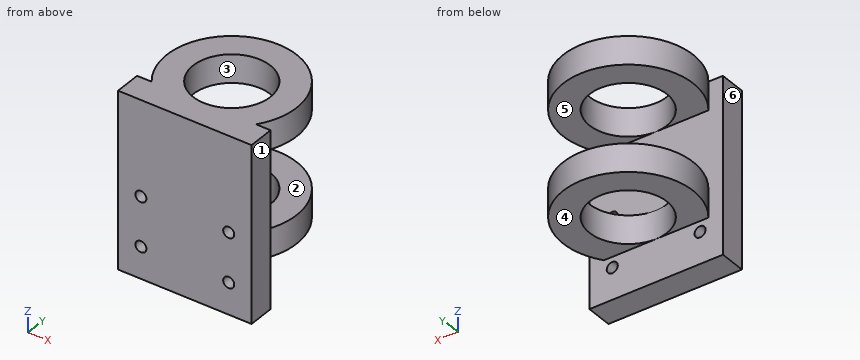
```python
from build123d import *

# Parameters (mm, degrees)
ESQUISSE1_R                = 18.5
ESQUISSE1_R_2              = 11
BOSS_EXTRU_19_DEPTH        = 8
BOSS_EXTRU_20_DEPTH        = 30
BOSS_EXTRU_20_DEPTH_BACK   = 20
R_P_TITION_LIN_AIRE1_COUNT = 2
R_P_TITION_LIN_AIRE1_PITCH = 30
ENL_V_MAT_EXTRU_1_REACH    = 48.165
ESQUISSE8_R                = 1.575


with BuildPart() as part:
    # Esquisse1 → Boss.-Extru.19 (new body)
    with BuildSketch(Plane.XY):
        Circle(ESQUISSE1_R)
        Circle(ESQUISSE1_R_2, mode=Mode.SUBTRACT)
    boss_extru_19 = extrude(amount=-BOSS_EXTRU_19_DEPTH)

    # Esquisse1_5 → Boss.-Extru.20 (add, two sides: drawn at the far end of the back side and taken through both)
    with BuildSketch(Plane.XY.offset(-BOSS_EXTRU_20_DEPTH_BACK)):
        with BuildLine():
            ThreePointArc((14.874474781, -11), (8.329165624, -16.518928537), (0, -18.5))
            Line((0, -18.5), (19, -18.5))
            Line((19, -18.5), (19, -11))
            Line((19, -11), (14.874474781, -11))
        make_face()
        with BuildLine():
            Line((-19, -18.5), (0, -18.5))
            ThreePointArc((0, -18.5), (-8.329165624, -16.518928537), (-14.874474781, -11))
            Line((-14.874474781, -11), (-19, -11))
            Line((-19, -11), (-19, -18.5))
        make_face()
        with BuildLine():
            Line((0, -11), (0, -11.058417443))
            Line((0, -11.058417443), (0, -18.5))
            ThreePointArc((0, -18.5), (8.329165624, -16.518928537), (14.874474781, -11))
            Line((14.874474781, -11), (1.4e-08, -11))
        make_face()
        with BuildLine():
            Line((0, -18.5), (0, -11.058417443))
            Line((0, -11.058417443), (0, -11))
            Line((1.4e-08, -11), (-14.874474781, -11))
            ThreePointArc((-14.874474781, -11), (-8.329165624, -16.518928537), (0, -18.5))
        make_face()
    extrude(amount=BOSS_EXTRU_20_DEPTH + BOSS_EXTRU_20_DEPTH_BACK)

    # R_p_tition lin_aire1: Boss.-Extru.19 ×2
    with Locations(*[(0, 0, i * R_P_TITION_LIN_AIRE1_PITCH) for i in range(1, R_P_TITION_LIN_AIRE1_COUNT)]):
        add(boss_extru_19)

    # Esquisse8 → Enl_v. mat.-Extru.1 (cut, up to next)
    with BuildSketch(Plane(origin=(0, -11, 0), x_dir=(1, 0, 0), z_dir=(0, 1, 0)), mode=Mode.PRIVATE) as enl_v_mat_extru_1_sk1:
        with Locations(Location((-12.5, 11, 0), (0, 0, 270))):
            Circle(ESQUISSE8_R)
    enl_v_mat_extru_1_tool1 = extrude(enl_v_mat_extru_1_sk1.sketch, amount=-ENL_V_MAT_EXTRU_1_REACH, mode=Mode.PRIVATE) & part.part
    # Esquisse8 → Enl_v. mat.-Extru.1 (cut, up to next)
    with BuildSketch(Plane(origin=(0, -11, 0), x_dir=(1, 0, 0), z_dir=(0, 1, 0)), mode=Mode.PRIVATE) as enl_v_mat_extru_1_sk2:
        with Locations(Location((12.5, 11, 0), (0, 0, 90))):
            Circle(ESQUISSE8_R)
    enl_v_mat_extru_1_tool2 = extrude(enl_v_mat_extru_1_sk2.sketch, amount=-ENL_V_MAT_EXTRU_1_REACH, mode=Mode.PRIVATE) & part.part
    # Esquisse8 → Enl_v. mat.-Extru.1 (cut, up to next)
    with BuildSketch(Plane(origin=(0, -11, 0), x_dir=(1, 0, 0), z_dir=(0, 1, 0)), mode=Mode.PRIVATE) as enl_v_mat_extru_1_sk3:
        with Locations(Location((12.5, -3, 0), (0, 0, 270))):
            Circle(ESQUISSE8_R)
    enl_v_mat_extru_1_tool3 = extrude(enl_v_mat_extru_1_sk3.sketch, amount=-ENL_V_MAT_EXTRU_1_REACH, mode=Mode.PRIVATE) & part.part
    # Esquisse8 → Enl_v. mat.-Extru.1 (cut, up to next)
    with BuildSketch(Plane(origin=(0, -11, 0), x_dir=(1, 0, 0), z_dir=(0, 1, 0)), mode=Mode.PRIVATE) as enl_v_mat_extru_1_sk4:
        with Locations(Location((-12.5, -3, 0), (0, 0, 90))):
            Circle(ESQUISSE8_R)
    enl_v_mat_extru_1_tool4 = extrude(enl_v_mat_extru_1_sk4.sketch, amount=-ENL_V_MAT_EXTRU_1_REACH, mode=Mode.PRIVATE) & part.part
    add(enl_v_mat_extru_1_tool1.solids().sort_by_distance((-12.5, -11, -11))[0], mode=Mode.SUBTRACT)
    add(enl_v_mat_extru_1_tool2.solids().sort_by_distance((12.5, -11, -11))[0], mode=Mode.SUBTRACT)
    add(enl_v_mat_extru_1_tool3.solids().sort_by_distance((12.5, -11, 3))[0], mode=Mode.SUBTRACT)
    add(enl_v_mat_extru_1_tool4.solids().sort_by_distance((-12.5, -11, 3))[0], mode=Mode.SUBTRACT)


solid = part.part
```
For this review, take the finished solid that the model builds, in its own axes (mm). Face numbers are marked on the shaded views. A direction names the side the tool comes from. Round coordinates to 2 decimals unless told otherwise and drop trailing zeros. Loops run counter-clockwise (first coordinate to the right, second up) from the corner with the lowest first, then second, coordinate; pieces in that order, holes last.
Q1. Mouldability with a two-part tool opening along X and no side actions: class the marked faces 1, 2 and 3 as +X half, -X half, draft (parallel to the pull), parting line (faces both ways), or undercut.
Result sheet:
face 1: +X half
face 2: draft
face 3: undercut
Q2. Add section A-A on y = 0. Write out the cut boundary in (x, z).
Result sheet:
outline: (-18.5, -8) - (-11, -8) - (-11, 0) - (-18.5, 0) - close; (-18.5, 22) - (-11, 22) - (-11, 30) - (-18.5, 30) - close; (11, -8) - (18.5, -8) - (18.5, 0) - (11, 0) - close; (11, 22) - (18.5, 22) - (18.5, 30) - (11, 30) - close
Q3. To check wall thickness, follow line 1 along X through (y, z) = (-12.75, 3) (3 decimals); line 2 along Z through (x, y) = (14.5, 4); line 3 along Z through (x, y) = (-12, -16). State the ranges of each line that lie inside material, in increasing order.
Result sheet:
line 1: x = -19 to -14.075, -10.925 to 10.925, 14.075 to 19
line 2: z = -8 to 0, 22 to 30
line 3: z = -20 to -12.49, -9.51 to 1.51, 4.49 to 30
Q4. Add section D-D on x = 12.5. Write out the cut boundary in (y, z) (3 decimals).
Result sheet:
outline: (-18.5, -20) - (-11, -20) - (-11, -12.575) - (-18.5, -12.575) - close; (-18.5, -9.425) - (-11, -9.425) - (-11, -8) - (13.638, -8) - (13.638, 0) - (-11, 0) - (-11, 1.425) - (-18.5, 1.425) - close; (-18.5, 4.575) - (-11, 4.575) - (-11, 22) - (13.638, 22) - (13.638, 30) - (-18.5, 30) - close
Q5. Machinability: for the marked faces 4, 5 and 6, which of the approach directions +Z, -Z, +X, -X, +Y, -Y give a long, thin tool a straight path to every point of the face, cutting with its end or side? Answer none if there is none.
Result sheet:
face 4: -Z, +X, -X, +Y
face 5: +X, -X, +Y
face 6: +Z, -Z, -X, +Y, -Y
Q6. Add section B-B on z = 3. Write out the cut boundary in (x, y) (3 decimals).
Result sheet:
outline: (-19, -18.5) - (-14.075, -18.5) - (-14.075, -11) - (-19, -11) - close; (-10.925, -18.5) - (10.925, -18.5) - (10.925, -11) - (-10.925, -11) - close; (14.075, -18.5) - (19, -18.5) - (19, -11) - (14.075, -11) - close
Q7. Insertion check: pin 1 Ø11.5 at (x, z) = (-9, -2.5) entering from +Y; pin 2 Ø20 at (x, y) = (0, 0) entering from -Z; pin 3 Ø5 at (x, y) = (3.5, 8) entering from -Z; pin 4 Ø8 at (y, z) = (13.5, 1) entering from -X. Each pin has a flat end and moves straight along its axis. Give the tip position at first contact, or say it passes through.
Result sheet:
pin 1: stops at y = 18.21
pin 2: passes through
pin 3: stops at z = -8
pin 4: stops at x = -15.8
Q8. Add section C-C on y = -14. Write out the cut boundary in (x, z) (3 decimals), plus the area to 3 significant figures.
Result sheet:
outline: (-19, -20) - (19, -20) - (19, 30) - (-19, 30) - close; hole circle Ø3.15 at (-12.5, -11); hole circle Ø3.15 at (-12.5, 3); hole circle Ø3.15 at (12.5, -11); hole circle Ø3.15 at (12.5, 3)
area: 1,870 mm2
